Autodesk Inventor part; units mm, degrees
ref_plane "YZ Plane" through (0, 0, 0) normal (1, 0, 0) x (0, 1, 0)
ref_plane "XZ Plane" through (0, 0, 0) normal (0, 1, 0) x (-1, 0, 0)
ref_plane "XY Plane" through (0, 0, 0) normal (0, 0, 1) x (1, 0, 0)
sketch "Sketch1" plane through (0, 0, 0) normal (0, 0, 1) x (1, 0, 0)
  circle A0 centre (0, 0) radius 2
  dimension "Diameter" = 4
extrude "Extrusion1" add sketch "Sketch1" along normal blind 16
sketch "Sketch2" plane through (0, 0, 16) normal (0, 0, 1) x (1, 0, 0)
  circle A0 centre (0, 0) radius 2
  circle A1 centre (0, 0) radius 3.5
  dimension "Head_Diameter" = 7
extrude "Extrusion2" add sketch "Sketch2" along normal blind 4 contours A0 | A1
sketch "Sketch3" plane through (0, 0, 20) normal (0, 0, 1) x (1, 0, 0)
  circle A0 centre (0, 0) radius 3.5
  circle A1 centre (0, 0) radius 1.7321 construction
  line L0 (0, 1.7321) -> (1.5, 0.866)
  line L1 (1.5, -0.866) -> (1.5, 0.866)
  line L2 (0, 1.7321) -> (-1.5, 0.866)
  line L3 (-1.5, -0.866) -> (-1.5, 0.866)
  line L4 (-1.5, -0.866) -> (0, -1.7321)
  line L5 (1.5, -0.866) -> (0, -1.7321)
  dimension "Hex_Width" = 3
extrude "Extrusion3" cut sketch "Sketch3" against normal blind 2 contours L0 L1 L5 L4 L3 L2
thread "Thread1"
chamfer "Chamfer1" distance 0.4 angle 45 2 edges at (-3.5, 0, 20) (-2, 0, 0)
equation "\"d9\" = ThreadLength"
equation "\"d12\" = Chamfer"
equation "\"ThreadLength\" = 20"
properties part number "SCREW, SOCKET HD, P, 12_9, M4X0_7X16" material "Steel, MS"
Source: CAD feature listing. Evaluate the final solid. Frame: model axes, mm. A direction names the side the tool comes from. Give positions to 0.01 mm unless a question says otherwise; leave off trailing zeros. Write each loop counter-clockwise with the first axis right and the second up, starting at its lowest first coordinate (ties: lowest second). Pieces come first, ordered by that corner, then holes. Notation, with made-up numbers: M 74.5,22.5 L 84.5,22.5 A14 cw 84.5,29.5 Z; hole C 25.25,51.5 d11. An arc over 180 degrees is marked long. Answer as a JSON object with one key per item and string values.
Q1. Access query for faces 1 (the face through (0.76, -1.293, 19.014)), 2 (the face through (0, 2, 8)), 3 (the face through (1.3, -1.3, 20)). Directions: +Z, -Z, +X, -X, +Y, -Y. A direction counts if a zero-diameter tool reaches every point of the face in a straight line with its end or side. Return the directions, or none.
Geometry check:
{"face 1": "+Z", "face 2": "-Z", "face 3": "+Z, +X, -X, +Y, -Y"}
Q2. Ray query, line 1 along Z through (x, y) = (0.75, -0.75); line 2 along Z through (x, y) = (-1.25, -2); line 3 along X through (y, z) = (-1, 3.5). Return the intervals inside material, ascending.
Geometry check:
{"line 1": "z = 0 to 18", "line 2": "z = 16 to 20", "line 3": "x = -1.73 to 1.73"}
Q3. Cut plane B-B, the plane z = 8.5. Return the cut outline in (x, y), then the cut area to 3 significant figures.
Geometry check:
{"outline": "C 0,0 d4", "area": "12.6 mm^2"}
Q4. Contact query for flat-ended pins moving along their axis: P1, Ø3, axis at x = 1.5, z = 6.5, coming from the +Y side; P2, Ø3, axis at y = 0, z = 7.5, coming from the +X side; P3, Ø0.9, axis at y = 0.5, z = 19, coming from the -X side; P4, Ø3, axis at y = 2, z = 4.5, coming from the +X side. Output: stop coordinate, or through.
Geometry check:
{"P1": "stops at y = 2", "P2": "stops at x = 2", "P3": "stops at x = -3.5", "P4": "stops at x = 1.94"}
Q5. Cut plane A-A, the plane y = 0. Return the cut outline in (x, z).
Geometry check:
{"outline": "M -3.5,16 L -2,16 L -2,0.4 L -1.6,0 L 1.6,0 L 2,0.4 L 2,16 L 3.5,16 L 3.5,19.6 L 3.1,20 L 1.5,20 L 1.5,18 L -1.5,18 L -1.5,20 L -3.1,20 L -3.5,19.6 Z"}
